Here's how the part is built. I have some questions about the finished solid (model axes, mm). A direction names the side the tool comes from. Coordinates: 2 decimals unless noted, no trailing zeros. Write each loop counter-clockwise with the first axis right and the second up, starting at its lowest first coordinate (ties: lowest second). Pieces come first, ordered by that corner, then holes. Notation, with made-up numbers: (38.5, 38.25) - (49.5, 38.25) arc R16 ccw to (49.5, 45.25) - close; hole circle Ø8 at (22, 33). An arc over 180 degrees is marked (long way). Answer in a Markdown table with one row per item. Add a question column.
Item 1: Which directions (+Z, -Z, +X, -X, +Y, -Y) give clear straight access to the entire face, cutting with the end or side of a thin tool? Please do faces 5 (the face through (-5.6, 16.9, 21.7)), 6 (the face through (5.6, 16.9, 28.3)), 7 (the face through (0, 17, 18.5)).
Item 2: Imagine slicing it at B-B (x = -1.25). Please give me the cut outline in (y, z).
Item 3: I'm going to push flat-ended pins straight in: pin 1 (3 mm diameter, centred on x = -3.5, y = -4.5, fed in from +Z); pin 2 (5 mm diameter, centred on x = 8.5, y = 15.5, fed in from +Z); pin 3 (2.5 mm diameter, centred on x = -1.5, y = 15.5, fed in from -Z). Where does each tip first touch, or does it pass through?
Item 4: Imagine slicing it at C-C (y = 8.5). Please give me the cut outline in (x, z) (3 decimals), plus the area to 3 significant figures.
Item 5: We'd pull the mould along Y, two halves only. Please class faces 1 (the face through (0, 0, 0)), 2 (the face through (-5.66, 16.92, 28.2)), 3 (the face through (0, 23, 25)), 4 (the face through (6, 0, -6)): +Y half, -Y half, draft (parallel to the pull), parting line (faces both ways), or undercut.
Item 6: If I drill on probe 1 along X at (y, z) = (-2, -5.5); probe 2 along Y at (x, z) = (-9.25, -5), over which ranges is the centre line in solid material (lowest first)? Write a range as from..to.
Item 7: Imagine slicing it at A-A (z = -5.5). Please give me the cut outline in (x, y).
Autodesk Fusion 360 part; units mm, degrees
sketch "Sketch1" plane through (0, 0, 0) normal (0, 0, 1) x (1, 0, 0)
  line L0 (6, 6) -> (-6, 6)
  line L1 (-6, 6) -> (-6, -6)
  line L2 (-6, -6) -> (6, -6)
  line L3 (6, -6) -> (6, 6)
  line L4 (6, 6) -> (-6, -6) construction
  line L5 (-6, 6) -> (6, -6) construction
  line L6 (-11, 11) -> (11, 11)
  line L7 (11, 11) -> (11, -11)
  line L8 (11, -11) -> (-11, -11)
  line L9 (-11, -11) -> (-11, 11)
  line L10 (-11, 11) -> (11, -11) construction
  line L11 (11, 11) -> (-11, -11) construction
  dimension "d1" = 12
  dimension "d2" = 12
  dimension "d3" = 5
extrude "Extrude1" add sketch "Sketch1" against normal blind 11.7 makes body 1
extrude "Extrude2" add sketch "Sketch1" along normal blind 2 contours L0 L1 L2 L3 | L6 L7 L8 L9 bodies 1
ref_plane "WorkPlane2" through (0, 11, 2) normal (0, 1, 0) x (-1, 0, 0)
sketch "Sketch3" plane through (0, 11, 0) normal (0, 1, 0) x (-1, 0, 0)
  line L0 (-3.7528, 31.5) -> (-7.5056, 25)
  line L1 (-7.5056, 25) -> (-3.7528, 18.5)
  line L2 (-3.7528, 18.5) -> (3.7528, 18.5)
  line L3 (3.7528, 18.5) -> (7.5056, 25)
  line L4 (7.5056, 25) -> (3.7528, 31.5)
  line L5 (3.7528, 31.5) -> (-3.7528, 31.5)
  line L6 (-11, 2) -> (11, 2)
  point P0 (0, 25)
  dimension "d10" = 13
  dimension "d19" = 16.5
extrude "Extrude4" add sketch "Sketch3" along normal blind 12 separate body makes body 2
extrude "Extrude7" add 1 faces at (-3.6667, 3.6667, 2) along direction (0, 0, 1) up to surface (29.5 mm away) on bodies 1 bodies 1 2
chamfer "Chamfer2" distance 30.765 distance2 4.087 2 edges at (11, 0, 31.5) (-11, 0, 31.5) measured on face at (11, 3.6667, 2.7) measured on face at (-11, -3.6667, 17.1) on bodies 1
chamfer "Chamfer2" distance 30.506 distance2 13.341 1 edges at (0, -11, 31.5) measured on face at (3.6667, -11, 2.7) on bodies 1
fillet "Fillet2" radius 3.625 2 edges at (8.9393, -4.3295, 16.247) (-8.9393, -4.3295, 16.247) on bodies 1
equation "d19 = ( ( 27 / 2 ) * 1 mm ) + 3 mm"
Here are the results:
| question | item | result |
|---|---|---|
| 1 | face 5 | -Z, -X, +Y |
| 1 | face 6 | +Z, +X, +Y |
| 1 | face 7 | -Z, +X, -X, +Y |
| 2 | outline | (-11, -11.7) - (-6, -11.7) - (-6, 0) - (6, 0) - (6, -11.7) - (11, -11.7) - (11, 18.5) - (23, 18.5) - (23, 31.5) - (2.34, 31.5) - (-11, 0.99) - close |
| 3 | pin 1 | stops at z = 19.29 |
| 3 | pin 2 | stops at z = 27.61 |
| 3 | pin 3 | stops at z = 18.5 |
| 4 | outline | (-11, -11.7) - (11, -11.7) - (11, 0.735) - (6.913, 31.5) - (-6.913, 31.5) - (-11, 0.735) - close |
| 4 | area | 825 mm2 |
| 5 | face 1 | undercut |
| 5 | face 2 | draft |
| 5 | face 3 | +Y half |
| 5 | face 4 | undercut |
| 6 | probe 1 | x = -11..-6, 6..11 |
| 6 | probe 2 | y = -11..11 |
| 7 | outline | (-11, -11) - (11, -11) - (11, 11) - (-11, 11) - close; hole (-6, -6) - (6, -6) - (6, 6) - (-6, 6) - close |
